Here's how the part is built. I have some questions about the finished solid (model axes, mm). Face numbers are marked on the shaded views. A direction names the side the tool comes from. Coordinates: 2 decimals unless noted, no trailing zeros. Write each loop counter-clockwise with the first axis right and the second up, starting at its lowest first coordinate (ties: lowest second). Pieces come first, ordered by that corner, then holes. Notation, with made-up numbers: (63, 55) -> (90, 55) arc R14 ccw to (90, 73) -> close; hole circle Ø2 at (-17.75, 16). An arc over 180 degrees is marked (long way). Answer in a Markdown table with one row per item. Add a question column.
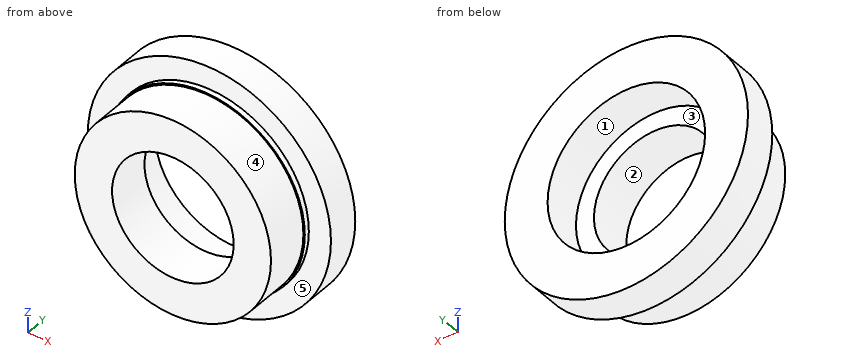
from build123d import *

# Parameters (mm, degrees)
SKETCH1_R           = 8.875
SKETCH1_R_2         = 5.5
BOSS_EXTRUDE1_DEPTH = 2
SKETCH2_R           = 9
SKETCH2_R_2         = 7.125
BOSS_EXTRUDE2_DEPTH = 3.5
SKETCH3_R           = 11
SKETCH3_R_2         = 9
BOSS_EXTRUDE3_DEPTH = 3


with BuildPart() as part:
    # Sketch1 → Boss-Extrude1 (new body, symmetric)
    with BuildSketch(Plane(origin=(0, 0, 0), x_dir=(1, 0, 0), z_dir=(0, 1, 0))):
        Circle(SKETCH1_R)
        Circle(SKETCH1_R_2, mode=Mode.SUBTRACT)
    extrude(amount=BOSS_EXTRUDE1_DEPTH, both=True)

    # Sketch2 → Boss-Extrude2 (add)
    with BuildSketch(Plane(origin=(0, 2, 0), x_dir=(1, 0, 0), z_dir=(0, 1, 0))):
        Circle(SKETCH2_R)
        Circle(SKETCH2_R_2, mode=Mode.SUBTRACT)
    extrude(amount=BOSS_EXTRUDE2_DEPTH)

    # Sketch3 → Boss-Extrude3 (add)
    with BuildSketch(Plane(origin=(0, 5.5, 0), x_dir=(1, 0, 0), z_dir=(0, 1, 0))):
        Circle(SKETCH3_R)
        Circle(SKETCH3_R_2, mode=Mode.SUBTRACT)
    extrude(amount=-BOSS_EXTRUDE3_DEPTH)


solid = part.part
Q1. For the marked faces 1 and 2, which set-ups out of +Z, -Z, +X, -X, +Y, -Y let a thin tool reach every point of the face, with its end or its side?
Q2. If we mould it in two halves opening along Z, with no side actions, what happens to the marked faces 3, 4 and 5? For each: pulls with the +Z half, pulls with the -Z half, needs draft (parallel to the pull), parting line crosses it, or undercut.
Q3. I'm going to push flat-ended pins straight in: P1, Ø1, axis at y = 1.5, z = -7, coming from the +X side; P2, Ø4.5, axis at x = 1, z = 1.5, coming from the +Y side. Where does each tip first touch, or does it pass through?
Q4. Imagine slicing it at B-B on x = 0. Please give me the cut outline in (y, z) (3 decimals), plus the area to 3 significant figures.
Q5. Imagine slicing it at A-A on z = 0. Please give me the cut outline in (x, y) (3 decimals), plus the area to 3 significant figures.
Q6. Imagine slicing it at D-D on z = -6. Please give me the cut outline in (x, y).
Q7. I need wall thicknesses on line 1 (X direction, y = -0.75, z = 0) (3 decimals); line 2 (X direction, y = 3.1, z = 0) (3 decimals). Which ranges of each line are inside material? Lowest first, please. Write a range as [from, to].
Q8. Imagine slicing it at C-C on y = -1. Please give me the cut outline in (x, z) (3 decimals).
Result sheet:
| question | item | result |
|---|---|---|
| 1 | face 1 | +Y |
| 1 | face 2 | +Y, -Y |
| 2 | face 3 | undercut |
| 2 | face 4 | parting line crosses it |
| 2 | face 5 | needs draft |
| 3 | P1 | stops at x = 6.04 |
| 3 | P2 | passes through |
| 4 | outline | (-2, -8.875) -> (2, -8.875) -> (2, -9) -> (2.5, -9) -> (2.5, -11) -> (5.5, -11) -> (5.5, -7.125) -> (2, -7.125) -> (2, -5.5) -> (-2, -5.5) -> close; (-2, 5.5) -> (2, 5.5) -> (2, 7.125) -> (5.5, 7.125) -> (5.5, 11) -> (2.5, 11) -> (2.5, 9) -> (2, 9) -> (2, 8.875) -> (-2, 8.875) -> close |
| 4 | area | 52.1 mm^2 |
| 5 | outline | (-11, 2.5) -> (-9, 2.5) -> (-9, 2) -> (-8.875, 2) -> (-8.875, -2) -> (-5.5, -2) -> (-5.5, 2) -> (-7.125, 2) -> (-7.125, 5.5) -> (-11, 5.5) -> close; (5.5, -2) -> (8.875, -2) -> (8.875, 2) -> (9, 2) -> (9, 2.5) -> (11, 2.5) -> (11, 5.5) -> (7.125, 5.5) -> (7.125, 2) -> (5.5, 2) -> close |
| 5 | area | 52.1 mm^2 |
| 6 | outline | (-9.22, 2.5) -> (-6.71, 2.5) -> (-6.71, 2) -> (-6.54, 2) -> (-6.54, -2) -> (6.54, -2) -> (6.54, 2) -> (6.71, 2) -> (6.71, 2.5) -> (9.22, 2.5) -> (9.22, 5.5) -> (3.84, 5.5) -> (3.84, 2) -> (-3.84, 2) -> (-3.84, 5.5) -> (-9.22, 5.5) -> close |
| 7 | line 1 | x = [-8.875, -5.5], [5.5, 8.875] |
| 7 | line 2 | x = [-11, -7.125], [7.125, 11] |
| 8 | outline | circle Ø17.75 at (0, 0); hole circle Ø11 at (0, 0) |
